Geometry check sheet. Reference: drawing and pictorial views, mm from the part's lowest x, y, z. Round coordinates to 2 decimals unless told otherwise and drop trailing zeros. Order: outer loops, then holes, each group sorted by start corner. A loop starts at its lowest first (then second) coordinate and runs counter-clockwise, first axis right, second up.
(1) Material ranges on line 1 along Z through (x, y) = (10, 2.5); line 2 along Z through (x, y) = (12.25, 3.25); line 3 along X through (y, z) = (1, 16.5), recorded low to high.
(2) Sectioned sample at C-C (z = 10). Record the boundary of the cut face in (x, y).
(3) Release check for a two-part mould opening along Z. For the marked faces 1, 2 and 3 record: +Z half, -Z half, draft (parallel to the pull), parting line (faces both ways), or undercut.
(4) Sectioned sample at B-B (x = 10). Record the boundary of the cut face in (y, z).
(5) Sectioned sample at A-A (y = 1). Record the boundary of the cut face in (x, z).
(6) Sectioned sample at D-D (x = 13.5). Record the boundary of the cut face in (y, z), plus the area to 3 significant figures.
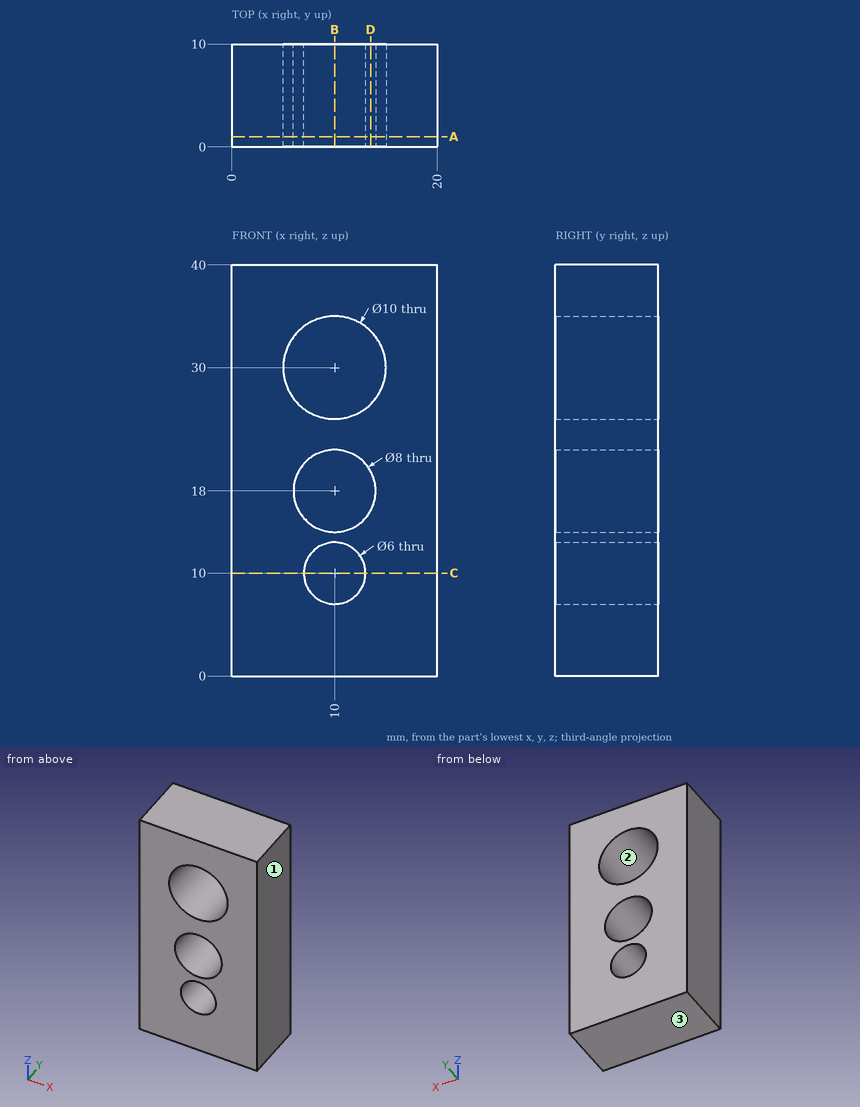
Answer below:
1. line 1: z = 0 to 7, 13 to 14, 22 to 25, 35 to 40
1. line 2: z = 0 to 8.02, 11.98 to 14.69, 21.31 to 25.53, 34.47 to 40
1. line 3: x = 0 to 6.29, 13.71 to 20
2. outline: (0, 0) - (7, 0) - (7, 10) - (0, 10) - close; (13, 0) - (20, 0) - (20, 10) - (13, 10) - close
3. face 1: draft
3. face 2: undercut
3. face 3: -Z half
4. outline: (0, 0) - (10, 0) - (10, 7) - (0, 7) - close; (0, 13) - (10, 13) - (10, 14) - (0, 14) - close; (0, 22) - (10, 22) - (10, 25) - (0, 25) - close; (0, 35) - (10, 35) - (10, 40) - (0, 40) - close
5. outline: (0, 0) - (20, 0) - (20, 40) - (0, 40) - close; hole circle Ø10 at (10, 30); hole circle Ø8 at (10, 18); hole circle Ø6 at (10, 10)
6. outline: (0, 0) - (10, 0) - (10, 16.06) - (0, 16.06) - close; (0, 19.94) - (10, 19.94) - (10, 26.43) - (0, 26.43) - close; (0, 33.57) - (10, 33.57) - (10, 40) - (0, 40) - close
6. area: 290 mm2
